Autodesk Inventor part; units mm, degrees
ref_plane "Work Plane1" through (19.05, -3.175, 0) normal (0, 1, 0) x (-1, 0, 0)
ref_plane "YZ Plane" through (0, 0, 0) normal (1, 0, 0) x (0, 1, 0)
ref_plane "XZ Plane" through (0, 0, 0) normal (0, 1, 0) x (-1, 0, 0)
sketch "Sketch1" plane through (0, 0, 0) normal (0, 0, 1) x (1, 0, 0)
  circle A0 centre (0, 0) radius 9.525 construction
  circle A1 centre (0, 0) radius 2.5527
  arc A2 (5.08, 3.81) -> (-5.08, 3.81) centre (0, 0) ccw
  arc A3 (5.08, 3.81) -> (19.05, -3.175) centre (19.05, 14.2875) ccw
  arc A4 (-19.05, -3.175) -> (-5.08, 3.81) centre (-19.05, 14.2875) ccw
  line L0 (-19.05, -9.525) -> (19.05, -9.525)
  line L1 (19.05, -9.525) -> (19.05, -3.175)
  line L2 (-19.05, -9.525) -> (-19.05, -3.175)
  dimension "d0" = 19.05
  dimension "d1" = 5.1054
  dimension "d2" = 12.7
  dimension "d3" = 6.35
  dimension "d4" = 38.1
extrude "Extrusion1" add sketch "Sketch1" along normal mid plane 25.4
ref_plane "Work Plane1" through (19.05, -3.175, 0) normal (0, 1, 0) x (-1, 0, 0)
sketch "Sketch2" plane through (19.05, -3.175, 0) normal (0, 1, 0) x (-1, 0, 0)
  line L0 (38.1, -12.7) -> (38.1, 12.7)
  line L1 (38.1, 0) -> (0, 0)
  line L2 (0, -12.7) -> (0, 12.7)
  circle A0 centre (31.75, 0) radius 2.4892
  circle A1 centre (31.75, 0) radius 5.2705
  circle A2 centre (6.35, 0) radius 5.2705
  circle A3 centre (6.35, 0) radius 2.4892
  point P0 (19.05, 0)
  dimension "d7" = 4.9784
  dimension "d8" = 10.541
  dimension "d11" = 360
  dimension "d13" = 25.4
extrude "Extrusion2" cut sketch "Sketch2" against normal through all contours A0 L1 | L1 A0 | A3 L1 | L1 A3
extrude "Extrusion3" cut sketch "Sketch2" along normal blind 25.4
fillet "Fillet1" radius 6.35 4 edges at (-19.05, -6.35, 12.7) (-19.05, -6.35, -12.7) (19.05, -6.35, 12.7) (19.05, -6.35, -12.7)
properties part number "254 Billet Thrust Block"
Here's how the part is built. I have some questions about the finished solid (model axes, mm). A direction names the side the tool comes from. Round coordinates to 2 decimals unless told otherwise and drop trailing zeros. Write each loop counter-clockwise with the first axis right and the second up, starting at its lowest first coordinate (ties: lowest second). Pieces come first, ordered by that corner, then holes.
1. Suppose I cut it at C-C (y = -6). List the corners of the cut face in (x, z) for me, and give its area (3 significant figures).
2. Suppose I cut it at D-D (y = 0). List the corners of the cut face in (x, z) for me, and give its area (3 significant figures).
3. For faces 1 (the cylindrical face through (-0.08, 6.35, -0.18)), 2 (the flat face through (10, -3.175, -1)), which set-ups out of +Z, -Z, +X, -X, +Y, -Y let a thin tool reach every point of the face, with its end or its side?
4. Suppose I cut it at B-B (z = 0). State how many separate pieces and enclosed holes the cut face has, and give its area (3 significant figures).
5. If we mould it in two halves opening along Y, with no side actions, what happens to faces 3 (the cylindrical face through (-10.213, -6.306, 0.109)), 4 (the cylindrical face through (6.941, 1.706, -0.178)), 5 (the cylindrical face through (2.435, -0.767, -0.178))? For each: released by +Y, released by -Y, zero draft, split by the parting line, or undercut.
6. Suppose I cut it at A-A (x = 0). List the corners of the cut face in (y, z) for me (3 decimals).
7. I need wall thicknesses on L1, parallel to X at y = -4.5, z = 0; L2, parallel to Z at x = -12.7, y = -5.5; L3, parallel to Z at x = 14.5, y = -5.75. Which ranges of each line are inside material? Lowest first, please.
8. Will these pins go through, and if not, where does the flat tip stop? pin 1 Ø1 at (x, y) = (-9.5, 2) entering from -Z; pin 2 Ø6.5 at (x, z) = (12.7, 0) entering from +Y (3 decimals); pin 3 Ø11.5 at (x, z) = (10, -0.5) entering from +Y; pin 4 Ø5 at (y, z) = (1, 7.5) entering from +X.
Answer sheet:
1. outline: (-19.05, -6.35) arc R6.35 ccw to (-12.7, -12.7) - (12.7, -12.7) arc R6.35 ccw to (19.05, -6.35) - (19.05, 6.35) arc R6.35 ccw to (12.7, 12.7) - (-12.7, 12.7) arc R6.35 ccw to (-19.05, 6.35) - close; hole circle Ø4.98 at (-12.7, 0); hole circle Ø4.98 at (12.7, 0)
1. area: 894 mm2
2. outline: (-9.01, -12.7) - (-2.55, -12.7) - (-2.55, 12.7) - (-9.01, 12.7) - (-9.01, 3.76) arc R5.27 cw to (-9.01, -3.76) - close; (2.55, -12.7) - (9.01, -12.7) - (9.01, -3.76) arc R5.27 cw to (9.01, 3.76) - (9.01, 12.7) - (2.55, 12.7) - close
2. area: 312 mm2
3. face 1: +Z, -Z, +Y
3. face 2: +Y
4. separate pieces: 3
4. enclosed holes: 1
4. area: 274 mm2
5. face 3: zero draft
5. face 4: released by +Y
5. face 5: undercut
6. outline: (-9.525, -12.7) - (-2.553, -12.7) - (-2.553, 12.7) - (-9.525, 12.7) - close; (2.553, -12.7) - (6.35, -12.7) - (6.35, 12.7) - (2.553, 12.7) - close
7. L1: x = -19.05 to -15.19, -10.21 to 10.21, 15.19 to 19.05
7. L2: z = -12.7 to -2.49, 2.49 to 12.7
7. L3: z = -12.44 to -1.72, 1.72 to 12.44
8. pin 1: passes through
8. pin 2: stops at y = -3.175
8. pin 3: stops at y = 4.72
8. pin 4: stops at x = 11.59
